Autodesk Inventor part; units mm, degrees
ref_plane "YZ Plane" through (0, 0, 0) normal (1, 0, 0) x (0, 1, 0)
ref_plane "XZ Plane" through (0, 0, 0) normal (0, 1, 0) x (-1, 0, 0)
ref_plane "XY Plane" through (0, 0, 0) normal (0, 0, 1) x (1, 0, 0)
sketch "Sketch1" plane through (0, 0, 0) normal (1, 0, 0) x (0, 1, 0)
  line L0 (0, 0) -> (0, -6)
  line L1 (0, -6) -> (13, -6)
  line L2 (0, 0) -> (3, 0)
  line L3 (3, 0) -> (3, 2)
  line L4 (3, 2) -> (1.1991, 2)
  line L5 (1.1991, 2) -> (-0.8009, 2)
  line L6 (-0.8009, 2) -> (-0.8009, -8)
  line L7 (-0.8009, -8) -> (14.1991, -8)
  line L8 (0, -3) -> (14.1991, -3)
  line L9 (14.1991, -8) -> (14.1991, -3)
  line L10 (13, -6) -> (13, -3)
  line L11 (14.1991, -3) -> (14.1991, 2)
  line L12 (14.1991, 2) -> (13, 2)
  line L13 (13, 2) -> (13, -3)
  line L14 (14.1991, -3) -> (13.349, -3)
  dimension "d0" = 6
  dimension "d1" = 13
  dimension "d2" = 2
  dimension "d3" = 2
  dimension "d4" = 10
  dimension "d5" = 15
  dimension "d6" = 5
extrude "Extrusion1" add sketch "Sketch1" along normal blind 4 contours L0 L1 L10 L8 L9 L7 L6 L5 L4 L3 L2 | L13 L12 L11 L8
sketch "Sketch3" plane through (0, 14.1991, 2) normal (0, 1, 0) x (1, 0, 0)
  line L0 (2, 1) -> (2.6492, 1)
  circle A0 centre (2, 1) radius 0.5
  point P0 (0, 2)
  dimension "d12" = 1
properties part number "Hook"
Here's how the part is built. I have some questions about the finished solid (model axes, mm). A direction names the side the tool comes from. Round coordinates to 2 decimals unless told otherwise and drop trailing zeros. Loops run counter-clockwise (first coordinate to the right, second up) from the corner with the lowest first, then second, coordinate; pieces in that order, holes last.
1. If we section it at A-A on z = 0.5: Write out the boundary of the cut face in (x, y), plus the area to 3 significant figures.
Answer list:
outline: (0, -0.8) - (4, -0.8) - (4, 3) - (0, 3) - close; (0, 13) - (4, 13) - (4, 14.2) - (0, 14.2) - close
area: 20.0 mm2
2. If we section it at B-B on y = 2.5: Write out the boundary of the cut face in (x, z), plus the area to 3 significant figures.
Answer list:
outline: (0, -8) - (4, -8) - (4, -6) - (0, -6) - close; (0, 0) - (4, 0) - (4, 2) - (0, 2) - close
area: 16.0 mm2
3. Which directions (+Z, -Z, +X, -X, +Y, -Y) give clear straight access to the entire face, cutting with the end or side of a thin tool? Please do faces 4 (the face through (2, -0.801, -3)), 5 (the face through (2, 1, 0)), 6 (the face through (2, 13, -2)).
Answer list:
face 4: +Z, -Z, +X, -X, -Y
face 5: +X, -X
face 6: +Z, +X, -X
4. If we section it at D-D on y = 7.5: Write out the boundary of the cut face in (x, z).
Answer list:
outline: (0, -8) - (4, -8) - (4, -6) - (0, -6) - close
5. We'd pull the mould along Y, two halves only. Please class faces 1 (the face through (2, 14.199, -3)), 2 (the face through (2, 6, -6)), 3 (the face through (2, 7, -8)): +Y half, -Y half, draft (parallel to the pull), parting line (faces both ways), or undercut.
Answer list:
face 1: +Y half
face 2: undercut
face 3: draft
6. If we section it at C-C on x = 2.4: Write out the boundary of the cut face in (y, z).
Answer list:
outline: (-0.8, -8) - (14.2, -8) - (14.2, 2) - (13, 2) - (13, -6) - (0, -6) - (0, 0) - (3, 0) - (3, 2) - (-0.8, 2) - close
7. If I drill on line 1 along Y through (x, z) = (0.95, -4.5); line 2 along Y through (x, z) = (1.2, 0.75); line 3 along Z through (x, y) = (0.75, 11.5), over which ranges is the centre line in solid material (lowest first)?
Answer list:
line 1: y = -0.8 to 0, 13 to 14.2
line 2: y = -0.8 to 3, 13 to 14.2
line 3: z = -8 to -6
